Study the drawing (mm; zero at the part's minimum x, y, z) and answer. Round coordinates to 2 decimals unless told otherwise and drop trailing zeros. Write each loop counter-clockwise with the first axis right and the second up, starting at its lowest first coordinate (ties: lowest second). Pieces come first, ordered by that corner, then holes.
(1) This flat-tipped pin is pushed along its axis until it touches: pin 1 Ø2.5 at (x, y) = (6.5, 34.5) entering from +Z. Where does it stop, or does it pass through?
(2) Find the intervals of material crossed by probe 1 along X at (y, z) = (30.5, 12.5); probe 2 along Z at (x, y) = (8, 62), in increasing order.
(3) A cutting plane is placed at B-B, the plane y = 15.5. Give the vertices of the cut face in (x, z).
(4) A cutting plane is placed at A-A, the plane z = 16.5. Give the vertices of the cut face in (x, y), and give its area (3 significant figures).
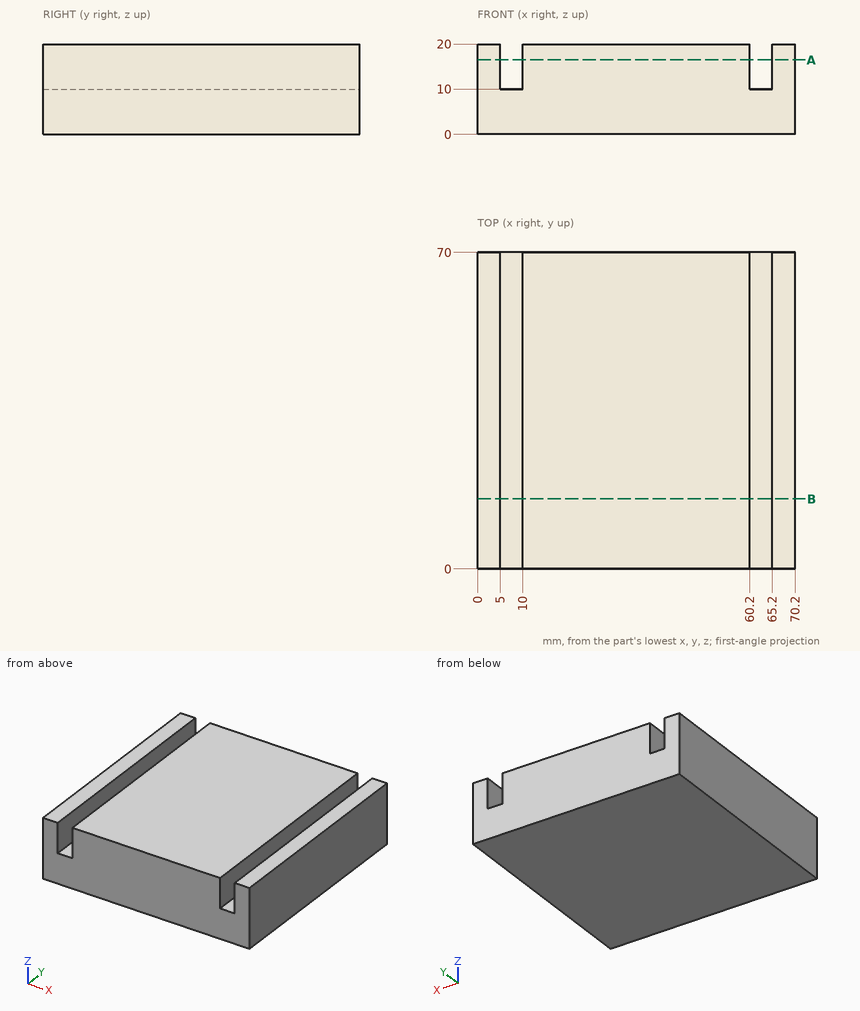
Solutions:
1. pin 1: stops at z = 10
2. probe 1: x = 0 to 5, 10 to 60.2, 65.2 to 70.2
2. probe 2: z = 0 to 10
3. outline: (0, 0) - (70.2, 0) - (70.2, 20) - (65.2, 20) - (65.2, 10) - (60.2, 10) - (60.2, 20) - (10, 20) - (10, 10) - (5, 10) - (5, 20) - (0, 20) - close
4. outline: (0, 0) - (5, 0) - (5, 70) - (0, 70) - close; (10, 0) - (60.2, 0) - (60.2, 70) - (10, 70) - close; (65.2, 0) - (70.2, 0) - (70.2, 70) - (65.2, 70) - close
4. area: 4,210 mm2
